from build123d import *

# Parameters (mm, degrees)
BOSS_EXTRU_1_DEPTH      = 39
ESQUISSE2_R             = 1.25
ENL_V_MAT_EXTRU_1_DEPTH = 39
ESQUISSE3_R             = 11
ESQUISSE3_R_2           = 4.6
BOSS_EXTRU_2_DEPTH      = 2
ESQUISSE4_R             = 2.5
BOSS_EXTRU_3_DEPTH      = 22.5
ESQUISSE5_W             = 9.5
ESQUISSE5_H             = 5
ENL_V_MAT_EXTRU_2_REACH = 83.969
ESQUISSE6_R             = 1.25
ENL_V_START             = -7
ENL_V_MAT_EXTRU_4_DEPTH = 7
ESQUISSE9_W             = 16
ESQUISSE9_H             = 10
BOSS_EXTRU_4_DEPTH      = 6.3


with BuildPart() as part:
    # Esquisse1 → Boss.-Extru.1 (new body)
    with BuildSketch(Plane(origin=(0, 0, 0), x_dir=(1, 0, 0), z_dir=(0, 1, 0))):
        Polygon((3.535533906, 2.549558154), (0, 6.08509206), (0, 41.014024248), (3.535533906, 44.549558154), (38.464466094, 44.549558154), (42, 41.014024248), (42, 6.08509206), (38.464466094, 2.549558154), align=None)
    extrude(amount=BOSS_EXTRU_1_DEPTH)

    # Esquisse2 → Enlèv. mat.-Extru.1 (cut)
    with BuildSketch(Plane(origin=(0, 39, 0), x_dir=(1, 0, 0), z_dir=(0, 1, 0))):
        with Locations(Location((5.3, 39.249558154, 0), (0, 0, 270))):
            Circle(ESQUISSE2_R)
        with Locations(Location((36.7, 39.249558154, 0), (0, 0, 270))):
            Circle(ESQUISSE2_R)
        with Locations(Location((36.7, 7.849558154, 0), (0, 0, 270))):
            Circle(ESQUISSE2_R)
        with Locations(Location((5.3, 7.849558154, 0), (0, 0, 270))):
            Circle(ESQUISSE2_R)
    extrude(amount=-ENL_V_MAT_EXTRU_1_DEPTH, mode=Mode.SUBTRACT)

    # Esquisse3 → Boss.-Extru.2 (add)
    with BuildSketch(Plane(origin=(0, 39, 0), x_dir=(1, 0, 0), z_dir=(0, 1, 0))):
        with Locations(Location((21, 23.549558154, 0), (0, 0, 90))):
            Circle(ESQUISSE3_R)
        with Locations(Location((21, 23.549558154, 0), (0, 0, 270))):
            Circle(ESQUISSE3_R_2, mode=Mode.SUBTRACT)
    extrude(amount=BOSS_EXTRU_2_DEPTH)

    # Esquisse4 → Boss.-Extru.3 (add)
    with BuildSketch(Plane(origin=(0, 39, 0), x_dir=(1, 0, 0), z_dir=(0, 1, 0))):
        with Locations(Location((21, 23.549558154, 0), (0, 0, 90))):
            Circle(ESQUISSE4_R)
    extrude(amount=BOSS_EXTRU_3_DEPTH)

    # Esquisse5 → Révolution1 (revolve)
    with BuildSketch(Plane(origin=(21, 0, 0), x_dir=(0, 0, -1), z_dir=(1, 0, 0)), mode=Mode.PRIVATE) as r_volution1_sk:
        with Locations((18.799558154, 52)):
            Rectangle(ESQUISSE5_W, ESQUISSE5_H)
    revolve(r_volution1_sk.sketch.rotate(Axis((21, 61.5, -23.549558154), (0, -1, 0)), 180), axis=Axis((21, 61.5, -23.549558154), (0, -1, 0)))

    # Esquisse6 → Enlèv. mat.-Extru.2 (cut, up to next)
    with BuildSketch(Plane(origin=(0, 54.5, 0), x_dir=(1, 0, 0), z_dir=(0, 1, 0)), mode=Mode.PRIVATE) as enl_v_mat_extru_2_sk1:
        with Locations(Location((27.3, 23.549558154, 0), (0, 0, 270))):
            Circle(ESQUISSE6_R)
    enl_v_mat_extru_2_tool1 = extrude(enl_v_mat_extru_2_sk1.sketch, amount=-ENL_V_MAT_EXTRU_2_REACH, mode=Mode.PRIVATE) & part.part
    # Esquisse6 → Enlèv. mat.-Extru.2 (cut, up to next)
    with BuildSketch(Plane(origin=(0, 54.5, 0), x_dir=(1, 0, 0), z_dir=(0, 1, 0)), mode=Mode.PRIVATE) as enl_v_mat_extru_2_sk2:
        with Locations(Location((21, 17.249558154, 0), (0, 0, 270))):
            Circle(ESQUISSE6_R)
    enl_v_mat_extru_2_tool2 = extrude(enl_v_mat_extru_2_sk2.sketch, amount=-ENL_V_MAT_EXTRU_2_REACH, mode=Mode.PRIVATE) & part.part
    # Esquisse6 → Enlèv. mat.-Extru.2 (cut, up to next)
    with BuildSketch(Plane(origin=(0, 54.5, 0), x_dir=(1, 0, 0), z_dir=(0, 1, 0)), mode=Mode.PRIVATE) as enl_v_mat_extru_2_sk3:
        with Locations(Location((14.7, 23.549558154, 0), (0, 0, 270))):
            Circle(ESQUISSE6_R)
    enl_v_mat_extru_2_tool3 = extrude(enl_v_mat_extru_2_sk3.sketch, amount=-ENL_V_MAT_EXTRU_2_REACH, mode=Mode.PRIVATE) & part.part
    # Esquisse6 → Enlèv. mat.-Extru.2 (cut, up to next)
    with BuildSketch(Plane(origin=(0, 54.5, 0), x_dir=(1, 0, 0), z_dir=(0, 1, 0)), mode=Mode.PRIVATE) as enl_v_mat_extru_2_sk4:
        with Locations(Location((21, 29.849558154, 0), (0, 0, 270))):
            Circle(ESQUISSE6_R)
    enl_v_mat_extru_2_tool4 = extrude(enl_v_mat_extru_2_sk4.sketch, amount=-ENL_V_MAT_EXTRU_2_REACH, mode=Mode.PRIVATE) & part.part
    add(enl_v_mat_extru_2_tool1.solids().sort_by_distance((27.3, 54.5, -23.549558))[0], mode=Mode.SUBTRACT)
    add(enl_v_mat_extru_2_tool2.solids().sort_by_distance((21, 54.5, -17.249558))[0], mode=Mode.SUBTRACT)
    add(enl_v_mat_extru_2_tool3.solids().sort_by_distance((14.7, 54.5, -23.549558))[0], mode=Mode.SUBTRACT)
    add(enl_v_mat_extru_2_tool4.solids().sort_by_distance((21, 54.5, -29.849558))[0], mode=Mode.SUBTRACT)

    # Esquisse8 → Enlèv. mat.-Extru.4 (cut)
    with BuildSketch(Plane(origin=(0, 61.5, 0), x_dir=(1, 0, 0), z_dir=(0, 1, 0)).offset(ENL_V_START)):
        with BuildLine():
            Line((22.47490916, 21.530983664), (19.52509084, 21.530983664))
            ThreePointArc((19.52509084, 21.530983664), (21, 21.049558154), (22.47490916, 21.530983664))
        make_face()
    extrude(amount=ENL_V_MAT_EXTRU_4_DEPTH, mode=Mode.SUBTRACT)

    # Esquisse9 → Boss.-Extru.4 (add)
    with BuildSketch(Plane(origin=(42, 0, 0), x_dir=(0, 0, -1), z_dir=(1, 0, 0))):
        with Locations((23.549024248, 5)):
            Rectangle(ESQUISSE9_W, ESQUISSE9_H)
    extrude(amount=BOSS_EXTRU_4_DEPTH)


solid = part.part
Source: CAD feature listing. Evaluate the final solid. Frame: model axes, mm. A direction names the side the tool comes from. Round coordinates to 2 decimals unless told otherwise and drop trailing zeros. Loops run counter-clockwise (first coordinate to the right, second up) from the corner with the lowest first, then second, coordinate; pieces in that order, holes last. Notation, with made-up numbers: M 60.25,16 L 116.25,16 A9 cw 116.25,25 Z; hole C -36,77 d1. An arc over 180 degrees is marked long. Answer as CSV lines item,"result".
Q1. Cut plane A-A (x = 36.7). Return the cut outline in (y, z), plus the area to 3 significant figures.
Verdict:
outline,"M 0,-44.55 L 39,-44.55 L 39,-40.5 L 0,-40.5 Z; M 0,-38 L 39,-38 L 39,-9.1 L 0,-9.1 Z; M 0,-6.6 L 39,-6.6 L 39,-2.55 L 0,-2.55 Z"
area,"1,440 mm^2"
Q2. Pull-direction query (Y, two-part tool) for faces 5 (the face through (17.361, 52.035, -32.325)), 6 (the face through (24.88, 39.99, -21.08)), 7 (the face through (21, 54.5, -21)); classes: +Y half, -Y half, draft (parallel to the pull), parting line (faces both ways), or undercut.
Verdict:
face 5,"draft"
face 6,"undercut"
face 7,"+Y half"
Q3. Line query: line 1 along Y through (x, z) = (17, -29); line 2 along X through (y, z) = (21, -8); line 3 along Z through (x, y) = (37.5, 27). Output: solid intervals per line, ascending.
Verdict:
line 1,"y = 0 to 41, 49.5 to 54.5"
line 2,"x = 0 to 4.06, 6.54 to 35.46, 37.94 to 42"
line 3,"z = -44.55 to -40.21, -38.29 to -8.81, -6.89 to -2.55"
Q4. Cut plane C-C (z = -8). Return the cut outline in (x, y).
Verdict:
outline,"M 0,0 L 4.06,0 L 4.06,39 L 0,39 Z; M 6.54,0 L 35.46,0 L 35.46,39 L 6.54,39 Z; M 37.94,0 L 42,0 L 42,39 L 37.94,39 Z"
Q5. Cut plane D-D (x = 21). Count the separate pieces of the cut face and the enclosed holes in it, plus the area to 3 significant figures.
Verdict:
separate pieces,"3"
enclosed holes,"0"
area,"1,820 mm^2"
Q6. Cut plane B-B (y = 25). Return the cut outline in (x, z), plus the area to 3 significant figures.
Verdict:
outline,"M 0,-41.01 L 3.54,-44.55 L 38.46,-44.55 L 42,-41.01 L 42,-6.09 L 38.46,-2.55 L 3.54,-2.55 L 0,-6.09 Z; hole C 5.3,-39.25 d2.5; hole C 5.3,-7.85 d2.5; hole C 36.7,-39.25 d2.5; hole C 36.7,-7.85 d2.5"
area,"1,720 mm^2"
Q7. Reachability of faces 1 (the face through (31.738, 39.986, -21.165)), 2 (the face through (1.793, 19.227, -4.293)), 3 (the face through (19.31, 44.18, -21.71)), 4 (the face through (45, 5, -31.549)) from +Z, -Z, +X, -X, +Y, -Y: full face, straight path, thin tool, end or side. Return the list, or none.
Verdict:
face 1,"+Y"
face 2,"+Z, -X, +Y, -Y"
face 3,"none"
face 4,"-Z, +X, +Y, -Y"
Q8. Contact query for flat-ended pins moving along their axis: pin 1 (1.5 mm diameter, centred on x = 5.3, z = -7.85, fed in from -Y) (1 decimal); pin 2 (8 mm diameter, centred on y = 53, z = -33.5, fed in from +X); pin 3 (3 mm diameter, centred on x = 44, y = 4.5, fed in from -Z); pin 4 (2 mm diameter, centred on x = 21, z = -17.25, fed in from +Y). Output: stop coordinate, or through.
Verdict:
pin 1,"passes through"
pin 2,"stops at x = 28.41"
pin 3,"stops at z = -31.55"
pin 4,"stops at y = 41"
